Check sheet for the modelled part. Datum: model origin and axes. Units: mm. Give positions to 0.01 mm unless a question says otherwise; leave off trailing zeros. Write each loop counter-clockwise with the first axis right and the second up, starting at its lowest first coordinate (ties: lowest second). Pieces come first, ordered by that corner, then holes. Notation, with made-up numbers: (61, -32.5) -> (95, -32.5) arc R19 cw to (95, -8.5) -> close; hole circle Ø9 at (50, 59.5). An arc over 180 degrees is marked (long way). Answer as a JSON object with one key per item and string values.
from build123d import *

# Parameters (mm, degrees)
F0_W = 20
F0_H = 50
F2_T = -2
F4_D = 5.1054


with BuildPart() as f1:
    # F0 (on Front) → F1 (revolve)
    with BuildSketch(Plane.XZ):
        Rectangle(F0_W, F0_H)
    revolve(axis=Axis((10, 0, 0), (0, 0, 1)))

    # F2 (hollow: no face is removed)
    offset(amount=F2_T, mode=Mode.SUBTRACT)

    # F4 (through all)
    with Locations(Plane.XY.offset(25)):
        with Locations((10, 0)):
            Hole(F4_D / 2)


solid = f1.part
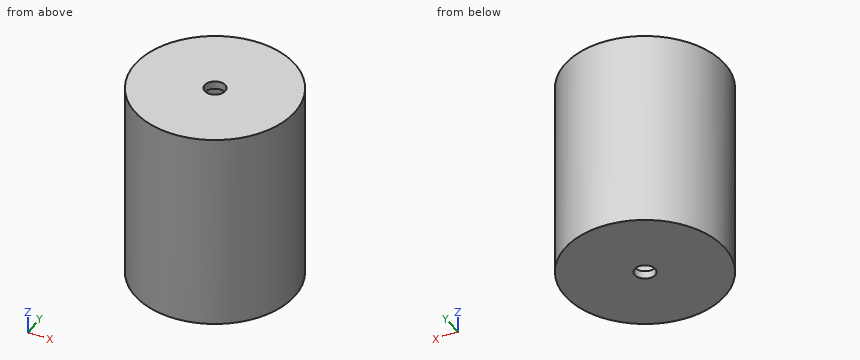
1. Sectioned sample at B-B, the plane x = 10. Enter the section's corners in (y, z), plus the area to 3 significant figures.
Determined:
{"outline": "(-20, -25) -> (-2.55, -25) -> (-2.55, -23) -> (-18, -23) -> (-18, 23) -> (-2.55, 23) -> (-2.55, 25) -> (-20, 25) -> close; (2.55, -25) -> (20, -25) -> (20, 25) -> (2.55, 25) -> (2.55, 23) -> (18, 23) -> (18, -23) -> (2.55, -23) -> close", "area": "324 mm^2"}
2. Go/stop test with flat-tipped pins: P1, Ø6, axis at x = 18.5, z = 9, coming from the +Y side; P2, Ø6, axis at x = 14.5, z = 12.5, coming from the +Y side; P3, Ø4, axis at x = 10, y = 0, coming from the -Z side; P4, Ø4, axis at y = 6.5, z = 5.5, coming from the +X side. Record where each tip stops, or that it passes through.
Determined:
{"P1": "y = 19.23", "P2": "y = 19.94", "P3": "through", "P4": "x = 29.49"}
3. Sectioned sample at D-D, the plane x = 24. Enter the section's corners in (y, z).
Determined:
{"outline": "(-14.28, -25) -> (14.28, -25) -> (14.28, 25) -> (-14.28, 25) -> close; hole (-11.31, -23) -> (11.31, -23) -> (11.31, 23) -> (-11.31, 23) -> close"}
4. Scan lines: L1, parallel to Z at x = 12, y = 3; L2, parallel to Y at x = 10, z = 23.75; L3, parallel to Y at x = 10, z = -15. Record each from-to range of solid material in increasing order. Write a range as [from, to].
Determined:
{"L1": "[-25, -23], [23, 25]", "L2": "[-20, -2.55], [2.55, 20]", "L3": "[-20, -18], [18, 20]"}
5. Sectioned sample at A-A, the plane y = 0. Enter the section's corners in (x, z).
Determined:
{"outline": "(-10, -25) -> (7.45, -25) -> (7.45, -23) -> (-8, -23) -> (-8, 23) -> (7.45, 23) -> (7.45, 25) -> (-10, 25) -> close; (12.55, -25) -> (30, -25) -> (30, 25) -> (12.55, 25) -> (12.55, 23) -> (28, 23) -> (28, -23) -> (12.55, -23) -> close"}
6. Sectioned sample at C-C, the plane z = 17. Enter the section's corners in (x, y), plus the area to 3 significant figures.
Determined:
{"outline": "circle Ø40 at (10, 0); hole circle Ø36 at (10, 0)", "area": "239 mm^2"}
